```python
from build123d import *

# Parameters (mm, degrees)
F0_W     = 85
F0_H     = 43
F0_R     = 6
F1_DEPTH = 40
F2_R     = 10
F3_DEPTH = 43.001
F4_R     = 16
F4_R_2   = 10
F5_DEPTH = 9
F6_R     = 16
F6_R_2   = 10
F7_DEPTH = 9


with BuildPart() as f1:
    # F0 (on Front) → F1 (new body)
    with BuildSketch(Plane.XZ):
        with Locations((42.5, 21.5)):
            Rectangle(F0_W, F0_H)
        with Locations((42.5, 21.5)):
            Circle(F0_R, mode=Mode.SUBTRACT)
    extrude(amount=F1_DEPTH)

    # F2 (on face) → F3 (cut, through all)
    with BuildSketch(Plane(origin=(0, 0, 0), x_dir=(1, 0, 0), z_dir=(0, 0, -1))):
        with Locations((20, 20)):
            Circle(F2_R)
        with Locations((65, 20)):
            Circle(F2_R)
    extrude(amount=-F3_DEPTH, mode=Mode.SUBTRACT)

    # F4 (on face) → F5 (cut)
    with BuildSketch(Plane(origin=(0, 0, 0), x_dir=(1, 0, 0), z_dir=(0, 0, -1))):
        with Locations((20, 20)):
            Circle(F4_R)
        with Locations((20, 20)):
            Circle(F4_R_2, mode=Mode.SUBTRACT)
        with Locations((65, 20)):
            Circle(F4_R)
        with Locations((65, 20)):
            Circle(F4_R_2, mode=Mode.SUBTRACT)
    extrude(amount=-F5_DEPTH, mode=Mode.SUBTRACT)

    # F6 (on face) → F7 (cut)
    with BuildSketch(Plane.XY.offset(43)):
        with Locations((20, -20)):
            Circle(F6_R)
        with Locations((20, -20)):
            Circle(F6_R_2, mode=Mode.SUBTRACT)
        with Locations((65, -20)):
            Circle(F6_R)
        with Locations((65, -20)):
            Circle(F6_R_2, mode=Mode.SUBTRACT)
    extrude(amount=-F7_DEPTH, mode=Mode.SUBTRACT)


solid = f1.part
```
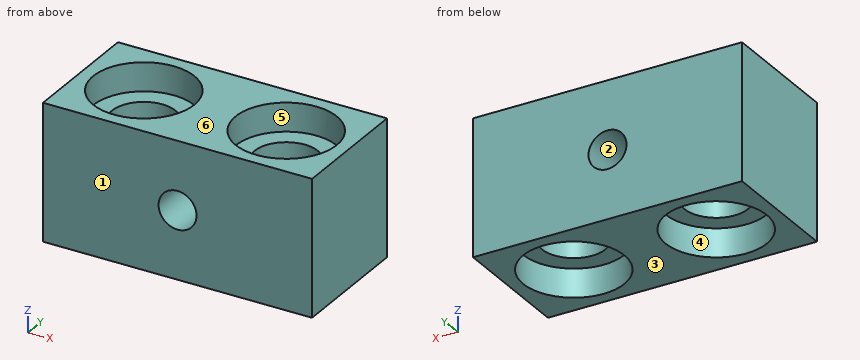
Input: part model. Units: mm. Frame: model coordinates. Face numbers are marked on the shaded views. A direction names the side the tool comes from. Give positions to 0.01 mm unless a question says otherwise; leave off trailing zeros. Order: outer loops, then holes, each group sorted by start corner. A loop starts at its lowest first (then second) coordinate and runs counter-clockwise, first axis right, second up. Notation, with made-up numbers: M 88.25,77.5 L 138.25,77.5 A26 ccw 138.25,91.5 Z; hole C 55.25,15 d1. An arc over 180 degrees is marked long. Return JSON: item names as keys, results as strings.
1) Section query B-B on x = 65. Output: boundary loops of the cut face in (y, z), and give its area (3 significant figures).
Taken from the geometry:
{"outline": "M -40,0 L -36,0 L -36,9 L -30,9 L -30,34 L -36,34 L -36,43 L -40,43 Z; M -10,9 L -4,9 L -4,0 L 0,0 L 0,43 L -4,43 L -4,34 L -10,34 Z", "area": "644 mm2"}
2) Line query: L1, parallel to X at y = -20, z = 4.75; L2, parallel to Y at x = 65, z = 5; L3, parallel to Y at x = 20, z = 18.75. Output: solid intervals per line, ascending. Write a range as [from, to].
Taken from the geometry:
{"L1": "x = [0, 4], [36, 49], [81, 85]", "L2": "y = [-40, -36], [-4, 0]", "L3": "y = [-40, -30], [-10, 0]"}
3) Mould query, pull axis Z, two halves, no side actions, for the marked faces 1, 2 and 3. Classes: released by +Z, released by -Z, zero draft, split by the parting line, or undercut.
Taken from the geometry:
{"face 1": "zero draft", "face 2": "undercut", "face 3": "released by -Z"}
4) Contact query for a flat-ended pin moving along its axis: pin 1 (16 mm diameter, centred on x = 67, y = -18, fed in from -Z). Output: stop coordinate, or through.
Taken from the geometry:
{"pin 1": "stops at z = 9"}
5) Section query A-A on y = -20. Count the separate pieces of the cut face and the enclosed holes in it, and give its area (3 significant figures).
Taken from the geometry:
{"separate pieces": "3", "enclosed holes": "1", "area": "1,390 mm2"}
6) Section query C-C on z = 25. Output: boundary loops of the cut face in (x, y), and give its area (3 significant figures).
Taken from the geometry:
{"outline": "M 0,-40 L 37.63,-40 L 37.63,0 L 0,0 Z; M 47.37,-40 L 85,-40 L 85,0 L 47.37,0 Z; hole C 20,-20 d20; hole C 65,-20 d20", "area": "2,380 mm2"}
7) Access query for the marked faces 4, 5 and 6. Directions: +Z, -Z, +X, -X, +Y, -Y. A direction counts if a zero-diameter tool reaches every point of the face in a straight line with its end or side. Return the directions, or none.
Taken from the geometry:
{"face 4": "-Z", "face 5": "+Z", "face 6": "+Z, +X, -X, +Y, -Y"}
8) Section query D-D on z = 40.5. Output: boundary loops of the cut face in (x, y), and give its area (3 significant figures).
Taken from the geometry:
{"outline": "M 0,-40 L 85,-40 L 85,0 L 0,0 Z; hole C 20,-20 d32; hole C 65,-20 d32", "area": "1,790 mm2"}
